from build123d import *

# Parameters (mm, degrees)
SKETCH1_W           = 65.35
SKETCH1_H           = 47.35
BOSS_EXTRUDE1_DEPTH = 3.175
SKETCH2_W           = 4.5
SKETCH2_H           = 3.175
SKETCH2_W_2         = 3.175
SKETCH2_H_2         = 10
SKETCH2_W_3         = 10
CUT_EXTRUDE1_DEPTH  = 4.175


with BuildPart() as part:
    # Sketch1 → Boss-Extrude1 (new body)
    with BuildSketch(Plane(origin=(0, 0, 0), x_dir=(1, 0, 0), z_dir=(0, 1, 0))):
        with Locations((32.675, 23.675)):
            Rectangle(SKETCH1_W, SKETCH1_H)
    extrude(amount=BOSS_EXTRUDE1_DEPTH)

    # Sketch2 → Cut-Extrude1 (cut, through all)
    with BuildSketch(Plane.XZ):
        with Locations((59.925, -45.7625)):
            Rectangle(SKETCH2_W, SKETCH2_H)
        Polygon((65.35, -38.675), (62.175, -38.675), (62.175, -44.175), (62.175, -47.35), (65.35, -47.35), align=None)
        with Locations((63.7625, -23.675)):
            Rectangle(SKETCH2_W_2, SKETCH2_H_2)
        Polygon((62.175, -8.675), (65.35, -8.675), (65.35, 0), (62.175, 0), (62.175, -3.175), align=None)
        with Locations((59.925, -1.5875)):
            Rectangle(SKETCH2_W, SKETCH2_H)
        with Locations((42.675, -1.5875)):
            Rectangle(SKETCH2_W_3, SKETCH2_H)
        with Locations((42.675, -45.7625)):
            Rectangle(SKETCH2_W_3, SKETCH2_H)
        with Locations((22.675, -45.7625)):
            Rectangle(SKETCH2_W_3, SKETCH2_H)
        with Locations((5.425, -45.7625)):
            Rectangle(SKETCH2_W, SKETCH2_H)
        Polygon((0, -47.35), (3.175, -47.35), (3.175, -44.175), (3.175, -38.675), (0, -38.675), align=None)
        with Locations((1.5875, -23.675)):
            Rectangle(SKETCH2_W_2, SKETCH2_H_2)
        Polygon((3.175, -3.175), (3.175, 0), (0, 0), (0, -8.675), (3.175, -8.675), align=None)
        with Locations((5.425, -1.5875)):
            Rectangle(SKETCH2_W, SKETCH2_H)
        with Locations((22.675, -1.5875)):
            Rectangle(SKETCH2_W_3, SKETCH2_H)
    extrude(amount=-CUT_EXTRUDE1_DEPTH, mode=Mode.SUBTRACT)


solid = part.part
Part model, mm, in its own coordinate system. A direction names the side the tool comes from. Coordinates: 2 decimals unless noted, no trailing zeros. Loops run counter-clockwise (first coordinate to the right, second up) from the corner with the lowest first, then second, coordinate; pieces in that order, holes last. Notation, with made-up numbers: M -4.75,59.5 L 20.25,59.5 A11 cw 20.25,65.5 Z; hole C 53,20.25 d6. An arc over 180 degrees is marked long. Use a Markdown table: item, result. Add a question column.
Q1. Cut at A-A (z = -42). Write the cut outline in (x, y) (3 decimals), and give its area (3 significant figures).
Q2. Probe L1, parallel to X at y = 2.05, z = -6 (3 decimals); L2, parallel to Z at x = 20.5, y = 1.6 (3 decimals). List the from-to ranges inside material, lowest first.
Q3. Cut at B-B (x = 61). Write the cut outline in (y, z) (3 decimals).
Q4. Which spindle directions (+Z, -Z, +X, -X, +Y, -Y) get a long thin tool onto all of the face, cutting with end or side? Do faces 1 (the flat face through (27.675, 2, -46)), 2 (the flat face through (47.675, 2, -2)), 3 (the flat face through (2, 2, -38.675)). Say none if no direction does.
Q5. Pin check, flat tips, straight feed: P1, Ø1.5, axis at y = 1, z = -16.5, coming from the -X side; P2, Ø1.6, axis at y = 1, z = -7, coming from the -X side (3 decimals); P3, Ø1.6, axis at x = 23.5, y = 1, coming from the -Z side (3 decimals); P4, Ø1, axis at y = 2, z = -1.5, coming from the +X side (3 decimals). Stop position of each tip, or through.
Worked out:
| question | item | result |
|---|---|---|
| 1 | outline | M 3.175,0 L 62.175,0 L 62.175,3.175 L 3.175,3.175 Z |
| 1 | area | 187 mm2 |
| 2 | L1 | x = 3.175 to 62.175 |
| 2 | L2 | z = -44.175 to -3.175 |
| 3 | outline | M 0,-44.175 L 3.175,-44.175 L 3.175,-3.175 L 0,-3.175 Z |
| 4 | face 1 | -Z, +Y, -Y |
| 4 | face 2 | +Z, +Y, -Y |
| 4 | face 3 | -Z, -X, +Y, -Y |
| 5 | P1 | stops at x = 0 |
| 5 | P2 | stops at x = 3.175 |
| 5 | P3 | stops at z = -44.175 |
| 5 | P4 | stops at x = 57.675 |
